Source: CAD feature listing. Evaluate the final solid. Frame: model axes, mm. Coordinates: 2 decimals unless noted, no trailing zeros. Order: outer loops, then holes, each group sorted by start corner. A loop starts at its lowest first (then second) coordinate and runs counter-clockwise, first axis right, second up. Notation, with made-up numbers: (13.5, 4) - (54.5, 4) arc R17 cw to (54.5, 35) - close; hole circle Ø1 at (-34.75, -12.75). An arc over 180 degrees is marked (long way). One line per question, with ' | ' between items. Start each with the question number.
(1) Section C-C (x = -3). Return the cut outline in (y, z), then the cut area to 3 significant figures.
(2) Line query: line 1 along Y through (x, z) = (33.5, 0.7); line 2 along Z through (x, y) = (-1.5, -31.5). Output: solid intervals per line, ascending.
(3) Section A-A (y = 0). Return the cut outline in (x, z), then the cut area to 3 significant figures.
(4) Draft query along Y for faces 1 (the cylindrical face through (33.981, -45.424, 1.521)), 2 (the flat face through (0, 1, 3)), 3 (the flat face through (0, 46, 1)). Return one class per face: +Y half, -Y half, draft (parallel to the pull), parting line (faces both ways), or undercut.
(5) Section B-B (y = -35.5). Return the cut outline in (x, z), then the cut area to 3 significant figures.
(6) Contact query for flat-ended pins moving along their axis: P1, Ø12, axis at x = 12, y = -25, coming from the -Z side; P2, Ø1.2, axis at x = 33.5, y = 44.5, coming from the +Z side. Output: stop coordinate, or through.
from build123d import *

# Parameters (mm, degrees)
BOSS_EXTRUDE1_DEPTH       = 3
TAP_DRILL_FOR_3_56_TAP1_D = 2.0828
CUT_EXTRUDE1_DEPTH        = 0.1


with BuildPart() as part:
    # Sketch1 → Boss-Extrude1 (new body)
    with BuildSketch(Plane.XY):
        with BuildLine():
            Line((-33.5, 46), (33.5, 46))
            ThreePointArc((33.5, 46), (34.560660172, 45.560660172), (35, 44.5))
            Line((35, 44.5), (35, -44.5))
            ThreePointArc((35, -44.5), (34.560660172, -45.560660172), (33.5, -46))
            Line((33.5, -46), (-33.5, -46))
            ThreePointArc((-33.5, -46), (-34.560660172, -45.560660172), (-35, -44.5))
            Line((-35, -44.5), (-35, 44.5))
            ThreePointArc((-35, 44.5), (-34.560660172, 45.560660172), (-33.5, 46))
        make_face()
    extrude(amount=BOSS_EXTRUDE1_DEPTH)

    # Tap Drill for #3-56 Tap1 (through all)
    with Locations(Plane(origin=(0, 0, 0), x_dir=(-1, 0, 0), z_dir=(0, 0, -1))):
        with Locations((-33.5, 44.5), (33.5, -44.5), (33.5, 0), (-33.5, 0), (-33.5, -44.5), (33.5, 44.5)):
            Hole(TAP_DRILL_FOR_3_56_TAP1_D / 2)

    # Sketch7 → Cut-Extrude1 (cut)
    with BuildSketch(Plane(origin=(0, 0, 0), x_dir=(-1, 0, 0), z_dir=(0, 0, -1))):
        with BuildLine():
            Line((26, 44), (-28, 44))
            ThreePointArc((-28, 44), (-28.707106781, 43.707106781), (-29, 43))
            Line((-29, 43), (-29, -45))
            ThreePointArc((-29, -45), (-28.707106781, -45.707106781), (-28, -46))
            Line((-28, -46), (26, -46))
            ThreePointArc((26, -46), (26.707106781, -45.707106781), (27, -45))
            Line((27, -45), (27, 43))
            ThreePointArc((27, 43), (26.707106781, 43.707106781), (26, 44))
        make_face()
    extrude(amount=-CUT_EXTRUDE1_DEPTH, mode=Mode.SUBTRACT)


solid = part.part
Response values:
1) outline: (-46, 0.1) - (44, 0.1) - (44, 0) - (46, 0) - (46, 3) - (-46, 3) - close | area: 267 mm²
2) line 1: y = -46 to -45.54, -43.46 to -1.04, 1.04 to 43.46, 45.54 to 46 | line 2: z = 0.1 to 3
3) outline: (-35, 0) - (-34.54, 0) - (-34.54, 3) - (-35, 3) - close; (-32.46, 0) - (-27, 0) - (-27, 0.1) - (29, 0.1) - (29, 0) - (32.46, 0) - (32.46, 3) - (-32.46, 3) - close; (34.54, 0) - (35, 0) - (35, 3) - (34.54, 3) - close | area: 192 mm²
4) face 1: undercut | face 2: draft | face 3: +Y half
5) outline: (-35, 0) - (-27, 0) - (-27, 0.1) - (29, 0.1) - (29, 0) - (35, 0) - (35, 3) - (-35, 3) - close | area: 204 mm²
6) P1: stops at z = 0.1 | P2: passes through
